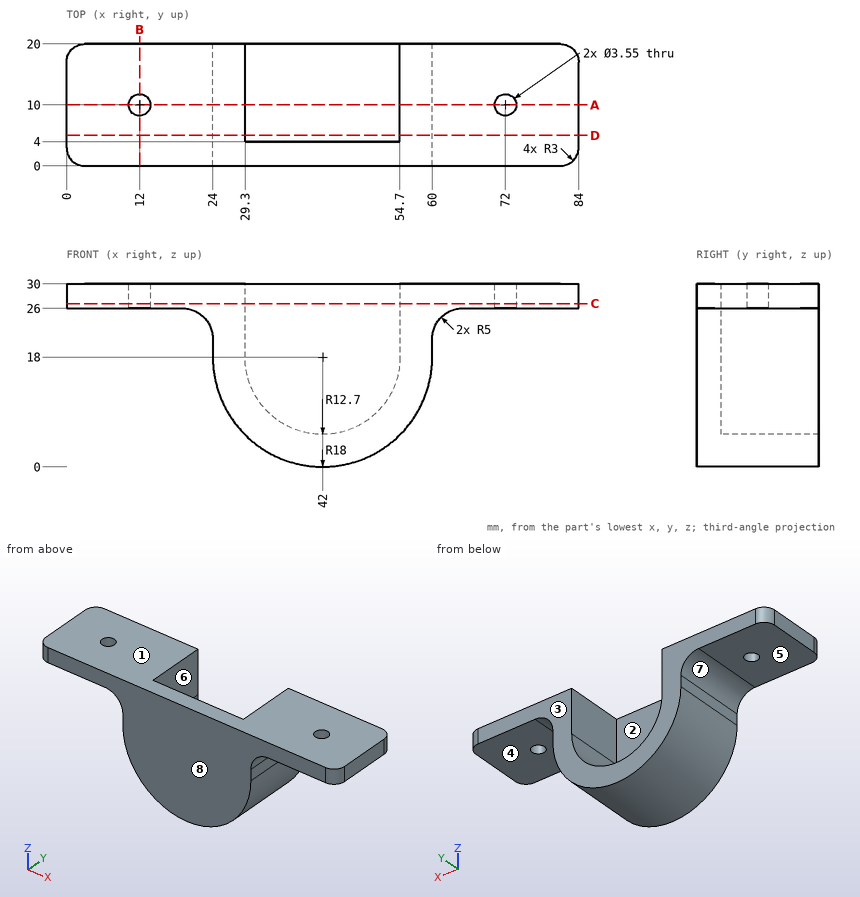
Part print with two shaded views. Sizes in mm from the minimum x, y, z corner. A direction names the side the tool comes from. Give positions to 0.01 mm unless a question says otherwise; leave off trailing zeros. Order: outer loops, then holes, each group sorted by start corner. A loop starts at its lowest first (then second) coordinate and runs counter-clockwise, first axis right, second up. Notation, with made-up numbers: M -38.5,63.5 L 13.5,63.5 A6 ccw 13.5,72.5 Z; hole C 24,11 d8. An arc over 180 degrees is marked long. Put each result on its own line as item: value.
Item 1: Cut at C-C on z = 26.75. Write the cut outline in (x, y) (3 decimals), then the cut area to 3 significant figures.
Results are:
outline: M 0,3 A3 ccw 3,0 L 81,0 A3 ccw 84,3 L 84,17 A3 ccw 81,20 L 54.7,20 L 54.7,4 L 29.3,4 L 29.3,20 L 3,20 A3 ccw 0,17 Z; hole C 12,10 d3.55; hole C 72,10 d3.55
area: 1,250 mm2
Item 2: Which spindle directions (+Z, -Z, +X, -X, +Y, -Y) get a long thin tool onto all of the face, cutting with end or side? Do the marked faces 1, 2, 3, 4 and 5. Say none if no direction does.
Results are:
face 1: +Z, +X, -X, +Y, -Y
face 2: +Z, +Y
face 3: +Z, -Z, +X, -X, +Y
face 4: -Z, +X, +Y, -Y
face 5: -Z, -X, +Y, -Y
Item 3: Drop flat-ended pins along their axis: pin 1 Ø5 at (y, z) = (17.5, 27) entering from +X; pin 2 Ø1.5 at (y, z) = (16, 16.5) entering from -X; pin 3 Ø9.5 at (x, y) = (72, 12) entering from -Z; pin 4 Ø2.5 at (y, z) = (7, 20) entering from +X. Give the stop position or say it passes through.
Results are:
pin 1: x = 84
pin 2: x = 24.02
pin 3: z = 26
pin 4: x = 60.01
Item 4: Cut at A-A on y = 10. Write the cut outline in (x, z) (3 decimals), then the cut area to 3 significant figures.
Results are:
outline: M 0,26 L 10.225,26 L 10.225,30 L 0,30 Z; M 13.775,26 L 19,26 A5 cw 24,21 L 24,18 A18 ccw 60,18 L 60,21 A5 cw 65,26 L 70.225,26 L 70.225,30 L 54.7,30 L 54.7,18 A12.7 cw 29.3,18 L 29.3,30 L 13.775,30 Z; M 73.775,26 L 84,26 L 84,30 L 73.775,30 Z
area: 557 mm2
Item 5: Pull direction X, two halves, no side cores. Call the marked faces 6, 7 and 8: +X half, -X half, draft (parallel to the pull), parting line (faces both ways), or undercut.
Results are:
face 6: undercut
face 7: -X half
face 8: draft
Item 6: Cut at D-D on y = 5. Write the cut outline in (x, z).
Results are:
outline: M 0,26 L 19,26 A5 cw 24,21 L 24,18 A18 ccw 60,18 L 60,21 A5 cw 65,26 L 84,26 L 84,30 L 54.7,30 L 54.7,18 A12.7 cw 29.3,18 L 29.3,30 L 0,30 Z
Item 7: Wall check: probe 1 along X at (y, z) = (17.5, 28.5); probe 2 along X at (y, z) = (14.25, 11); probe 3 along Y at (x, z) = (12, 28.4) (3 decimals). Give the ranges that are in metal, low to high.
Results are:
probe 1: 0.04 to 29.3, 54.7 to 83.96
probe 2: 25.42 to 31.4, 52.6 to 58.58
probe 3: 0 to 8.225, 11.775 to 20
Item 8: Cut at B-B on x = 12. Write the cut outline in (y, z) (3 decimals), then the cut area to 3 significant figures.
Results are:
outline: M 0,26 L 8.225,26 L 8.225,30 L 0,30 Z; M 11.775,26 L 20,26 L 20,30 L 11.775,30 Z
area: 65.8 mm2
